Autodesk Inventor part; units mm, degrees
ref_plane "YZ Plane" through (0, 0, 0) normal (1, 0, 0) x (0, 1, 0)
ref_plane "XZ Plane" through (0, 0, 0) normal (0, 1, 0) x (-1, 0, 0)
ref_plane "XY Plane" through (0, 0, 0) normal (0, 0, 1) x (1, 0, 0)
sketch "Sketch1" plane through (0, 0, 0) normal (0, 1, 0) x (-1, 0, 0)
  point P0 (0, 0)
sketch "Sketch2" plane through (0, 0, 0) normal (0, 1, 0) x (-1, 0, 0)
  line L0 (0, 0) -> (150, 0)
  line L1 (150, 0) -> (150, -150)
  line L2 (150, -150) -> (0, -150)
  line L3 (0, -150) -> (0, 0)
  dimension "d0" = 150
  dimension "d1" = 150
extrude "Extrusion1" add sketch "Sketch2" along normal blind 7.5
sketch "Sketch4" plane through (0, 7.5, 0) normal (0, 1, 0) x (1, 0, 0)
  line L0 (0, 0) -> (-150, 0)
  line L1 (0, 150) -> (0, 0)
  line L2 (-150, 0) -> (0, 0)
  line L3 (0, 0) -> (0, 150)
  line L4 (0, 150) -> (-150, 150)
  line L5 (-150, 150) -> (-150, 0)
  line L6 (-146, 4) -> (-4, 4)
  line L7 (-4, 4) -> (-4, 146)
  line L8 (-4, 146) -> (-146, 146)
  line L9 (-146, 146) -> (-146, 4)
  dimension "d7" = 4
extrude "Extrusion3" add sketch "Sketch4" along normal blind 35
sketch "Sketch5" plane through (0, 7.5, 0) normal (0, 1, 0) x (1, 0, 0)
  line L0 (-146, 146) -> (-146, 4)
  line L1 (-146, 4) -> (-136, 4)
  line L2 (-136, 4) -> (-136, 14)
  line L3 (-136, 14) -> (-146, 14)
  line L4 (-146, 14) -> (-146, 4)
  point P0 (0, 0)
  dimension "d10" = 10
  dimension "d11" = 10
extrude "Extrusion4" add sketch "Sketch5" along normal blind 35
pattern_linear "Rectangular Pattern1" count 2 spacing 132 along (0, 0, -1) count 2 spacing 132 along (1, 0, 0) of "Extrusion4"
sketch "Sketch6" plane through (0, 42.5, 0) normal (0, 1, 0) x (1, 0, 0)
  line L0 (-136, 14) -> (-146, 14)
  line L1 (-141, 14) -> (-141, 0)
  line L2 (0, 0) -> (-150, 0)
  circle A0 centre (-141, 9) radius 2.75
  dimension "d20" = 5.5
extrude "Extrusion5" cut sketch "Sketch6" against normal blind 80
pattern_linear "Rectangular Pattern2" count 2 spacing 132 along (0, 0, -1) count 2 spacing 132 along (1, 0, 0) of "Extrusion5"
sketch "Sketch9" plane through (0, 42.5, 0) normal (0, 1, 0) x (1, 0, 0)
  point P0 (0, 0)
sketch "Sketch10" plane through (0, 42.5, 0) normal (0, 1, 0) x (1, 0, 0)
  line L0 (-150, 150) -> (0, 150)
  line L1 (0, 0) -> (-150, 0)
  line L2 (0, 150) -> (-150, 150)
  line L3 (-150, 150) -> (-150, 0)
  line L4 (-150, 0) -> (0, 0)
  line L5 (0, 0) -> (0, 150)
  line L6 (-4, 146) -> (-146, 146)
  line L7 (-146, 146) -> (-146, 4)
  line L8 (-146, 4) -> (-4, 4)
  line L9 (-4, 4) -> (-4, 146)
  dimension "d45" = 4
extrude "Extrusion8" add sketch "Sketch10" along normal blind 40
sketch "Sketch11" plane through (0, 7.5, 0) normal (0, 1, 0) x (1, 0, 0)
  point P0 (0, 0)
properties part number "Bottom1"
Input: part model. Units: mm. Frame: model coordinates. A direction names the side the tool comes from. Give positions to 0.01 mm unless a question says otherwise; leave off trailing zeros. Order: outer loops, then holes, each group sorted by start corner. A loop starts at its lowest first (then second) coordinate and runs counter-clockwise, first axis right, second up.
1. Cut plane B-B (z = -9). Return loops of the section in (x, y).
Computed:
outline: (-150, 0) - (-143.75, 0) - (-143.75, 42.5) - (-146, 42.5) - (-146, 82.5) - (-150, 82.5) - close; (-138.25, 0) - (-11.75, 0) - (-11.75, 42.5) - (-14, 42.5) - (-14, 7.5) - (-136, 7.5) - (-136, 42.5) - (-138.25, 42.5) - close; (-6.25, 0) - (0, 0) - (0, 82.5) - (-4, 82.5) - (-4, 42.5) - (-6.25, 42.5) - close
2. Set-up query: faces 1 (the face through (-138.46, 21.55, -139.95)), 2 (the face through (-14, 25, -9)). Return all of +Z, -Z, +X, -X, +Y, -Y with unobstructed straight access to the full face (end or side cutting, diameter ignored); none if empty.
Computed:
face 1: +Y, -Y
face 2: +Y
3. Line query: probe 1 along X at (y, z) = (11.5, -9); probe 2 along X at (y, z) = (77, -24). Output: solid intervals per line, ascending.
Computed:
probe 1: x = -150 to -143.75, -138.25 to -136, -14 to -11.75, -6.25 to 0
probe 2: x = -150 to -146, -4 to 0
4. Cut plane D-D (y = 21). Return loops of the section in (x, z), and give its area (3 significant figures).
Computed:
outline: (-150, -150) - (0, -150) - (0, 0) - (-150, 0) - close; hole (-146, -136) - (-136, -136) - (-136, -146) - (-14, -146) - (-14, -136) - (-4, -136) - (-4, -14) - (-14, -14) - (-14, -4) - (-136, -4) - (-136, -14) - (-146, -14) - close; hole circle Ø5.5 at (-141, -141); hole circle Ø5.5 at (-141, -9); hole circle Ø5.5 at (-9, -141); hole circle Ø5.5 at (-9, -9)
area: 2,640 mm2
5. Draft query along X for faces 3 (the face through (-7.73, 21.55, -138.56)), 4 (the face through (-74, 41, 0)), 5 (the face through (-150, 41, -76)). Return one class per face: released by +X, released by -X, zero draft, split by the parting line, or undercut.
Computed:
face 3: undercut
face 4: zero draft
face 5: released by -X
6. Cut plane C-C (y = 59.5). Return loops of the section in (x, z), and give its area (3 significant figures).
Computed:
outline: (-150, -150) - (0, -150) - (0, 0) - (-150, 0) - close; hole (-146, -146) - (-4, -146) - (-4, -4) - (-146, -4) - close
area: 2,340 mm2
7. Pin query (flat end, axial travel): pin 1 Ø5 at (x, z) = (-9, -9) entering from +Y; pin 2 Ø12 at (x, z) = (-28.5, -68.5) entering from +Y. Return the tip coordinate at first contact, or that it passes through.
Computed:
pin 1: passes through
pin 2: stops at y = 7.5
8. Cut plane A-A (x = -141). Return loops of the section in (y, z), and give its area (3 significant figures).
Computed:
outline: (0, -150) - (82.5, -150) - (82.5, -146) - (42.5, -146) - (42.5, -143.75) - (0, -143.75) - close; (0, -138.25) - (42.5, -138.25) - (42.5, -136) - (7.5, -136) - (7.5, -14) - (42.5, -14) - (42.5, -11.75) - (0, -11.75) - close; (0, -6.25) - (42.5, -6.25) - (42.5, -4) - (82.5, -4) - (82.5, 0) - (0, 0) - close
area: 1,960 mm2
